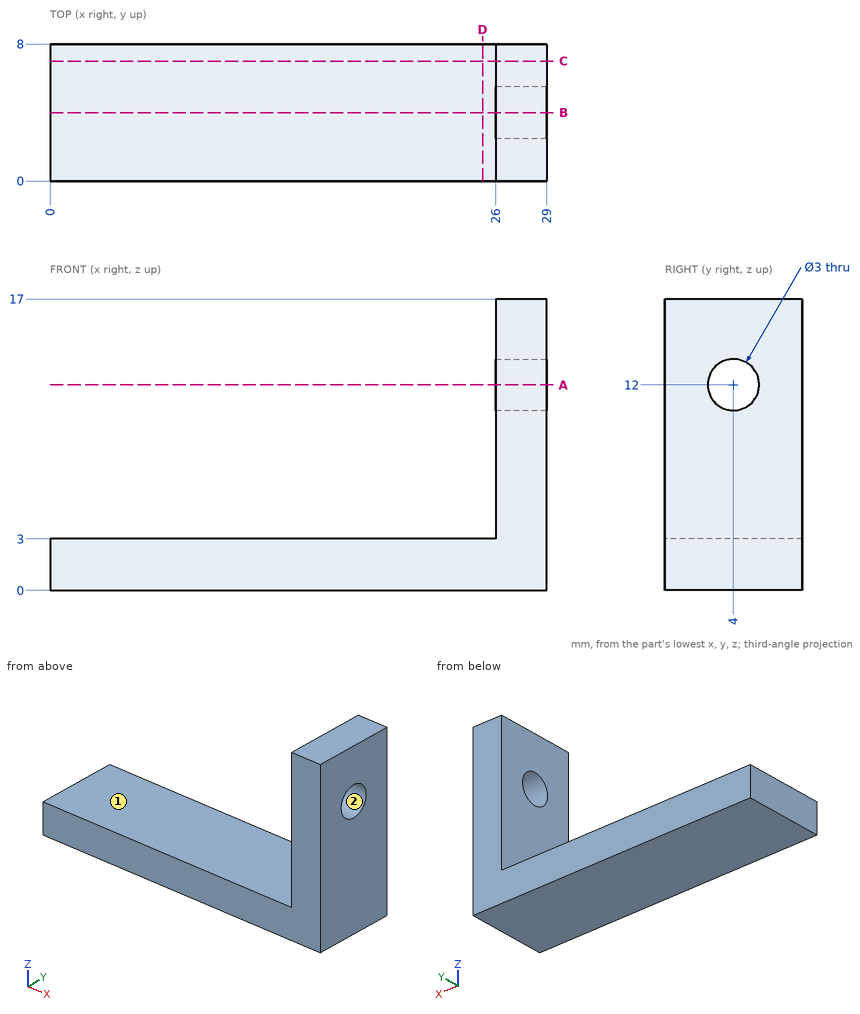
Here's the drawing with two shaded views (mm, measured from the low corner). I have some questions. A direction names the side the tool comes from. Give positions to 0.01 mm unless a question says otherwise; leave off trailing zeros. Order: outer loops, then holes, each group sorted by start corner. A loop starts at its lowest first (then second) coordinate and runs counter-clockwise, first axis right, second up. Notation, with made-up numbers: M 9,6 L 54,6 A33 cw 54,40 Z; hole C -32.5,67.25 d2. An arc over 180 degrees is marked long. One line per question, with ' | ' between items.
Item 1: Suppose I cut it at B-B, the plane y = 4. Write out the boundary of the cut face in (x, z).
Answer block:
outline: M 0,0 L 29,0 L 29,10.5 L 26,10.5 L 26,3 L 0,3 Z; M 26,13.5 L 29,13.5 L 29,17 L 26,17 Z
Item 2: Suppose I cut it at D-D, the plane x = 25.25. Write out the boundary of the cut face in (y, z).
Answer block:
outline: M 0,0 L 8,0 L 8,3 L 0,3 Z
Item 3: Suppose I cut it at C-C, the plane y = 7. Write out the boundary of the cut face in (x, z).
Answer block:
outline: M 0,0 L 29,0 L 29,17 L 26,17 L 26,3 L 0,3 Z
Item 4: Suppose I cut it at A-A, the plane z = 12. Write out the boundary of the cut face in (x, y).
Answer block:
outline: M 26,0 L 29,0 L 29,2.5 L 26,2.5 Z; M 26,5.5 L 29,5.5 L 29,8 L 26,8 Z
Item 5: I'm going to push flat-ended pins straight in: pin 1 Ø1.8 at (y, z) = (4, 12) entering from +X (3 decimals); pin 2 Ø2 at (y, z) = (6.5, 12) entering from -X; pin 3 Ø4 at (x, y) = (9.5, 3) entering from +Z. Where does each tip first touch, or does it pass through?
Answer block:
pin 1: passes through | pin 2: stops at x = 26 | pin 3: stops at z = 3
Item 6: Please list where these lines run through material, in increasing order: L1, parallel to Z at x = 28.25, y = 4; L2, parallel to Z at x = 7, y = 2.25; L3, parallel to X at y = 5.75, z = 7.75.
Answer block:
L1: z = 0 to 10.5, 13.5 to 17 | L2: z = 0 to 3 | L3: x = 26 to 29
Item 7: For the marked faces 1 and 2, which set-ups out of +Z, -Z, +X, -X, +Y, -Y let a thin tool reach every point of the face, with its end or its side?
Answer block:
face 1: +Z, -X, +Y, -Y | face 2: +X, -X
